Could you check a few things on this model? Use its own coordinates, in mm. Face numbers are marked on the shaded views. Give positions to 0.01 mm unless a question says otherwise; leave off trailing zeros. Write each loop counter-clockwise with the first axis right and the second up, starting at its lowest first coordinate (ties: lowest second). Pieces come first, ordered by that corner, then holes. Notation, with made-up numbers: M 57.5,70.5 L 83.5,70.5 A28 ccw 83.5,94.5 Z; hole C 5.25,16.25 d6. An arc over 180 degrees is marked long. Use one line per item in the form item = value.
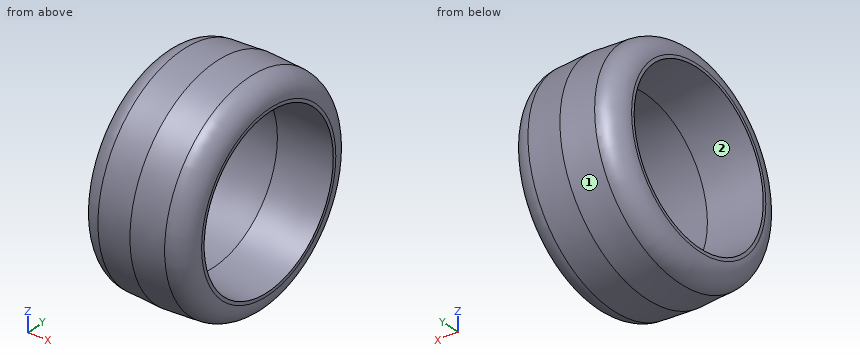
from build123d import *

# Parameters (mm, degrees)
F2_R     = 25.9753807736
F2_R_2   = 19.05
F3_DEPTH = 12.7
F3_TAPER = 3
F4_R     = 5.08


# Not quite as in the source:
# - two fillets or chamfers of one size are made in one step


with BuildPart() as f3:
    # F2 (on offset) → F3 (new body, symmetric)
    with BuildSketch(Plane.YZ.offset(50.8)):
        Circle(F2_R)
        Circle(F2_R_2, mode=Mode.SUBTRACT)
    extrude(amount=F3_DEPTH, both=True, taper=F3_TAPER)

    # F4
    f4_edges = [f3.edges().sort_by_distance(p)[0] for p in [
        (63.5, -25.309802, 0),
        (38.1, -25.309802, 0),
    ]]
    fillet(f4_edges, radius=F4_R)


solid = f3.part
1) If I drill on L1, parallel to Z at x = 48, y = -4; L2, parallel to Z at x = 43.5, y = 15.5; L3, parallel to Y at x = 47, z = 14, over which ranges is the centre line in solid material (lowest first)?
Checked values:
L1 = -25.52 to -18.78, 18.78 to 25.52
L2 = -20.37 to -11.72, 11.72 to 20.37
L3 = -21.64 to -13.21, 13.21 to 21.64
2) For pin 1 Ø1.5 at (x, z) = (50, -13.5) entering from -Y; pin 2 Ø1.5 at (x, y) = (60.5, 12.5) entering from +Z; pin 3 Ø8 at (x, z) = (59.5, -9) entering from -Y, each with a flat end and sliding along its axis, tell me the tip position at first contact or that it passes through.
Checked values:
pin_1 = -22.59
pin_2 = 22.33
pin_3 = -25.05
3) I want a section at C-C, the plane x = 44.75. Please give me the cut outline in (y, z).
Checked values:
outline = C 0,0 d51.32; hole C 0,0 d38.73
4) I want a section at B-B, the plane x = 58. Please give me the cut outline in (y, z), plus the area to 3 significant figures.
Checked values:
outline = C 0,0 d51.2; hole C 0,0 d38.85
area = 873 mm2
5) Thinking about a two-plate mould opening in Y: for the marked faces 1 and 2, which applies, released by +Y, released by -Y, zero draft, split by the parting line, or undercut?
Checked values:
face_1 = split by the parting line
face_2 = undercut
6) I want a section at A-A, the plane y = 0. Please give me the cut outline in (x, z).
Checked values:
outline = M 38.1,-20.49 A5.08 ccw 42.91,-25.56 L 50.8,-25.98 L 58.69,-25.56 A5.08 ccw 63.5,-20.49 L 63.5,-19.72 L 50.8,-19.05 L 38.1,-19.72 Z; M 38.1,19.72 L 50.8,19.05 L 63.5,19.72 L 63.5,20.49 A5.08 ccw 58.69,25.56 L 50.8,25.98 L 42.91,25.56 A5.08 ccw 38.1,20.49 Z
